Source: CAD feature listing. Evaluate the final solid. Frame: model axes, mm. A direction names the side the tool comes from. Give positions to 0.01 mm unless a question says otherwise; leave off trailing zeros. Write each loop counter-clockwise with the first axis right and the second up, starting at its lowest first coordinate (ties: lowest second). Pieces come first, ordered by that corner, then holes. Notation, with made-up numbers: (39.5, 4) -> (58.5, 4) arc R21 ccw to (58.5, 28) -> close; hole circle Ø8 at (37, 45). An arc over 180 degrees is marked (long way). Write item = value, one per line.
Autodesk Inventor part; units mm, degrees
ref_plane "YZ Plane" through (0, 0, 0) normal (1, 0, 0) x (0, 1, 0)
ref_plane "XZ Plane" through (0, 0, 0) normal (0, 1, 0) x (-1, 0, 0)
ref_plane "XY Plane" through (0, 0, 0) normal (0, 0, 1) x (1, 0, 0)
sketch "Sketch1" plane through (0, 0, 0) normal (0, 0, 1) x (1, 0, 0)
  circle A0 centre (0, 0) radius 2
  circle A1 centre (0, 0) radius 3.5
  dimension "d0" = 7
  dimension "d1" = 4
extrude "Extrusion1" add sketch "Sketch1" along normal blind 18
extrude "Extrusion2" add sketch "Sketch1" along normal blind 23 contours A0
fillet "Fillet1" radius 1 1 edges at (-3.5, 0, 18)
fillet "Fillet2" radius 0.4 1 edges at (-2, 0, 23)
mirror "Mirror1" about plane through (0, 0, 0) normal (0, 0, 1) of "Extrusion1", "Extrusion2", "Fillet1", "Fillet2"
equation "\"d2\" = 0.5 * length"
equation "\"length\" = 36"
properties part number "SCAMI D-PA C-RAIL ROLLER"
(1) Section query C-C (z = 4). Return loops of the section in (x, y), plus the area to 3 significant figures.
Values follow:
outline = circle Ø7 at (0, 0)
area = 38.5 mm2
(2) First-contact query: pin 1 (4 mm diameter, centred on y = 1, z = 14, fed in from +X); pin 2 (1 mm diameter, centred on y = 2, z = 10, fed in from -X). Flat tips, straight axial feed; report the tip coordinate or a pass-through.
Values follow:
pin_1 = 3.5
pin_2 = -3.16
(3) Access query for faces 1 (the face through (3.233, -1.341, 0.238)), 2 (the face through (-1, 2, 18)), 3 (the face through (0, -2, -20)). Directions: +Z, -Z, +X, -X, +Y, -Y. A direction counts if a zero-diameter tool reaches every point of the face in a straight line with its end or side. Return the directions, or none.
Values follow:
face_1 = +Z, -Z
face_2 = +Z
face_3 = -Z
(4) Section query A-A (x = 0). Return loops of the section in (y, z), plus the area to 3 significant figures.
Values follow:
outline = (-3.5, -17) arc R1 ccw to (-2.5, -18) -> (-2, -18) -> (-2, -22.6) arc R0.4 ccw to (-1.6, -23) -> (1.6, -23) arc R0.4 ccw to (2, -22.6) -> (2, -18) -> (2.5, -18) arc R1 ccw to (3.5, -17) -> (3.5, 17) arc R1 ccw to (2.5, 18) -> (2, 18) -> (2, 22.6) arc R0.4 ccw to (1.6, 23) -> (-1.6, 23) arc R0.4 ccw to (-2, 22.6) -> (-2, 18) -> (-2.5, 18) arc R1 ccw to (-3.5, 17) -> close
area = 291 mm2
(5) Material intervals for line 1 (Z direction, x = -1, y = 2.25); line 2 (X direction, y = 0.25, z = 0.5); line 3 (X direction, y = 2, z = -11), sorted ascending.
Values follow:
line_1 = -18 to 18
line_2 = -3.49 to 3.49
line_3 = -2.87 to 2.87
